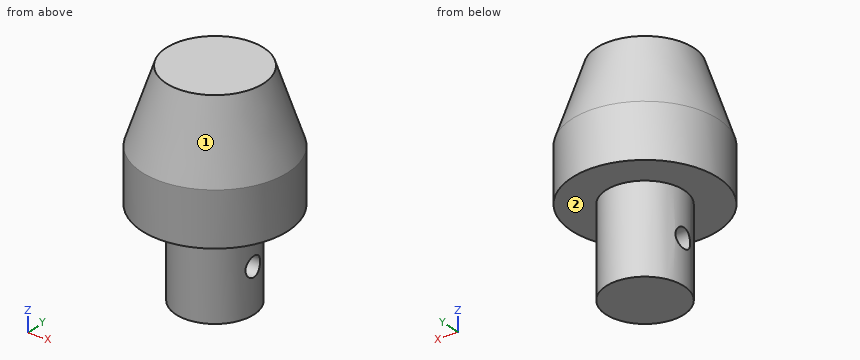
from build123d import *

# Parameters (mm, degrees)
SKETCH_2_R          = 2
CUT_EXTRUDE_1_DEPTH = 10


with BuildPart() as part:
    # 草圖1 → 旋轉1 (revolve)
    with BuildSketch(Plane(origin=(0, 0, 0), x_dir=(0, 0, -1), z_dir=(1, 0, 0))):
        Polygon((0, 0), (0, 10), (15, 15), (26, 15), (26, 8), (44, 8), (44, 0), align=None)
    revolve(axis=Axis((0, 0, -44), (0, 0, 1)))

    # 草圖2 → 除料-伸長1 (cut, symmetric)
    with BuildSketch(Plane(origin=(0, 0, 0), x_dir=(0, 0, -1), z_dir=(1, 0, 0))):
        with Locations((35, 0)):
            Circle(SKETCH_2_R)
    extrude(amount=CUT_EXTRUDE_1_DEPTH, both=True, mode=Mode.SUBTRACT)


solid = part.part
Part model, mm, in its own coordinate system. Face numbers are marked on the shaded views. A direction names the side the tool comes from. Coordinates: 2 decimals unless noted, no trailing zeros. Loops run counter-clockwise (first coordinate to the right, second up) from the corner with the lowest first, then second, coordinate; pieces in that order, holes last. Notation, with made-up numbers: (54.25, -15.5) - (75.25, -15.5) arc R10 cw to (75.25, 0.5) - close; hole circle Ø11 at (-5.5, 24). An arc over 180 degrees is marked (long way). Write each question's results on one line, items separated by ' | '. Start each with the question number.
Q1. Slice it at D-D on z = -30. Give the cut face in (x, y).
Q2. Drop flat-ended pins along their axis: pin 1 Ø8 at (x, y) = (-11.5, 3) entering from +Z; pin 2 Ø4.5 at (y, z) = (0, -35) entering from -X; pin 3 Ø6 at (y, z) = (2.5, -11) entering from -X; pin 4 Ø1.5 at (x, z) = (-12, -17) entering from +Y. Give the stop position or say it passes through.
Q3. Slice it at A-A on y = 0. Give the cut face in (x, z).
Q4. Slice it at C-C on z = -35. Give the cut face in (x, y), and give its area (3 significant figures).
Q5. Probe line 1 along Z through (x, y) = (9.5, -1.25); line 2 along Z through (x, y) = (4.5, 0); line 3 along Y through (x, z) = (-1.5, -35). List the from-to ranges inside material, lowest first.
Q6. Slice it at B-B on x = 0. Give the cut face in (y, z).
Q7. Which spindle directions (+Z, -Z, +X, -X, +Y, -Y) get a long thin tool onto all of the face, cutting with end or side? Do the marked faces 1 and 2. Say none if no direction does.
Answer:
1) outline: circle Ø16 at (0, 0)
2) pin 1: stops at z = 0 | pin 2: stops at x = -8 | pin 3: stops at x = -14.53 | pin 4: stops at y = 9.92
3) outline: (-15, -26) - (-8, -26) - (-8, -33) - (8, -33) - (8, -26) - (15, -26) - (15, -15) - (10, 0) - (-10, 0) - (-15, -15) - close; (-8, -44) - (8, -44) - (8, -37) - (-8, -37) - close
4) outline: (-7.75, -2) arc R8 ccw to (7.75, -2) - close; (-7.75, 2) - (7.75, 2) arc R8 ccw to start | area: 138 mm2
5) line 1: z = -26 to 0 | line 2: z = -44 to -37, -33 to 0 | line 3: y = -7.86 to -2, 2 to 7.86
6) outline: (-15, -26) - (-8, -26) - (-8, -44) - (8, -44) - (8, -26) - (15, -26) - (15, -15) - (10, 0) - (-10, 0) - (-15, -15) - close; hole circle Ø4 at (0, -35)
7) face 1: +Z | face 2: -Z
